Could you check a few things on this model? Use its own coordinates, in mm. A direction names the side the tool comes from. Round coordinates to 2 decimals unless told otherwise and drop trailing zeros. Loops run counter-clockwise (first coordinate to the right, second up) from the corner with the lowest first, then second, coordinate; pieces in that order, holes last. Notation, with made-up numbers: M 7.25,18 L 49.25,18 A15 ccw 49.25,47 Z; hole C -24.75,79.25 d2. An arc over 180 degrees is marked long. Answer in a Markdown table with one row per item.
Autodesk Inventor part; units mm, degrees
ref_plane "YZ Plane" through (0, 0, 0) normal (1, 0, 0) x (0, 1, 0)
ref_plane "XZ Plane" through (0, 0, 0) normal (0, 1, 0) x (-1, 0, 0)
ref_plane "XY Plane" through (0, 0, 0) normal (0, 0, 1) x (1, 0, 0)
sketch "Sketch1" plane through (0, 0, 0) normal (1, 0, 0) x (0, 1, 0)
  line L0 (0, 0) -> (73.993, 0)
  line L1 (0, 130.0359) -> (44.4227, 130.0359)
  line L2 (0, 130.0359) -> (0, 155.2107)
  line L3 (15.8613, 155.2107) -> (44.4227, 155.2107)
  line L4 (44.4227, 155.2107) -> (44.4227, 130.0359)
  line L5 (1.5875, 153.6232) -> (1.5875, 131.6234)
  line L6 (1.5875, 131.6234) -> (42.8352, 131.6234)
  line L7 (42.8352, 131.6234) -> (42.8352, 153.6232)
  line L8 (18.2426, 143.1015) -> (18.2426, 119.3292)
  line L9 (14.2738, 131.6234) -> (14.2738, 130.0359)
  line L10 (22.2113, 131.6234) -> (22.2113, 130.0359)
  line L11 (22.2113, 167.4765) -> (22.2113, 148.4065)
  line L12 (22.2113, 154.417) -> (28.5613, 154.417)
  line L13 (28.5613, 154.417) -> (28.5613, 153.6232)
  line L14 (22.2113, 154.417) -> (15.8613, 154.417)
  line L15 (15.8613, 154.417) -> (15.8613, 155.2107)
  line L16 (42.8352, 153.6232) -> (28.5613, 153.6232)
  line L17 (18.2426, 153.6232) -> (1.5875, 153.6232)
  dimension "d1" = 25.1748
  dimension "d2" = 130.0359
  dimension "d3" = 44.4227
  dimension "d4" = 0
  dimension "d5" = 1.5875
  dimension "d6" = 1.5875
  dimension "d7" = 1.5875
  dimension "d8" = 1.5875
  dimension "d9" = 18.2426
  dimension "d10" = 7.9375
  dimension "d11" = 3.9688
  dimension "d13" = 22.2113
  dimension "d15" = 6.35
  dimension "d16" = 6.35
revolve "Revolution1" add sketch "Sketch1" angle 90 about axis through (0, 0, 0) along (0, 1, 0) contours L10 L6 L7 L16 L13 L12 L11 L3 L4 L1 | L11 L14 L15 L3
equation "\"d2\" = 0.5 * IBDia - 3 * SpWall"
equation "\"d3\" = Wall + 4 * SpWall + BevDriverDia + d1_1"
equation "\"d5\" = Wall"
equation "\"d6\" = Wall"
equation "\"d7\" = Wall"
equation "\"d8\" = Wall"
equation "\"d9\" = 2 * SpWall + 0.5 * BevDriverDia"
equation "\"d10\" = AxelDia + Space"
equation "\"d11\" = 0.5 * Space + 0.5 * AxelDia"
equation "\"d13\" = 0.5 * d3"
equation "\"IDia\" = 266.7"
equation "\"Wall\" = 1.5875"
equation "\"Space\" = 1.5875"
equation "\"SpWall\" = 3.175"
equation "\"AxelDia\" = 6.35"
equation "\"d14\" = 0.5 * Wall"
properties part number "OuterShell_Top_Quarter"
1) I want a section at B-B, the plane x = 32. Please give me the cut outline in (y, z).
Computed:
| item | result |
|---|---|
| outline | M 15.86,151.06 L 28.56,151.06 L 28.56,150.25 L 42.84,150.25 L 42.84,127.67 L 22.21,127.67 L 22.21,126.04 L 44.42,126.04 L 44.42,151.88 L 15.86,151.88 Z |
2) I want a section at C-C, the plane z = 15. Please give me the cut outline in (x, y).
Computed:
| item | result |
|---|---|
| outline | M 129.17,22.21 L 130.77,22.21 L 130.77,42.84 L 152.89,42.84 L 152.89,28.56 L 153.69,28.56 L 153.69,15.86 L 154.48,15.86 L 154.48,44.42 L 129.17,44.42 Z |
3) Will these pins go through, and if not, where does the flat tip stop? P1, Ø2, axis at y = 33, z = 27, coming from the -X side; P2, Ø1.5, axis at y = 23.5, z = 77, coming from the +X side; P3, Ø8, axis at y = 20, z = 136.5, coming from the -X side.
Computed:
| item | result |
|---|---|
| P1 | stops at x = 126.99 |
| P2 | stops at x = 135.19 |
| P3 | stops at x = 64.07 |
4) I need wall thicknesses on line 1 (Y direction, x = 38, z = 131); line 2 (Z direction, x = 64, y = 29); line 3 (X direction, y = 27.5, z = 31.5). Which ranges of each line are inside material? Lowest first, please.
Computed:
| item | result |
|---|---|
| line 1 | y = 42.84 to 44.42 |
| line 2 | z = 113.2 to 115.02, 139.66 to 141.4 |
| line 3 | x = 126.16 to 127.8, 151.17 to 151.98 |
5) Which directions (+Z, -Z, +X, -X, +Y, -Y) give clear straight access to the entire face, cutting with the end or side of a thin tool? Please do faces 5 (the face through (109.816, 35.598, 107.427)), 6 (the face through (90.933, 33.472, 92.955)).
Computed:
| item | result |
|---|---|
| face 5 | -Y |
| face 6 | -Z, -X, +Y, -Y |
6) I want a section at A-A, the plane y = 24.5. Please give me the cut outline in (x, z), plus the area to 3 significant figures.
Computed:
| item | result |
|---|---|
| outline | M 0,130.04 A130.04 cw 130.04,0 L 131.62,0 A131.62 ccw 0,131.62 Z; M 0,154.42 A154.42 cw 154.42,0 L 155.21,0 A155.21 ccw 0,155.21 Z |
| area | 519 mm² |
7) If we mould it in two halves opening along X, with no side actions, what happens to faces 1 (the face through (0, 44, 144)), 2 (the face through (108.54, 30.34, 110.95)), 3 (the face through (107.982, 22.3, 110.383)), 4 (the face through (100, 22.211, 85))? For each: released by +X, released by -X, zero draft, split by the parting line, or undercut.
Computed:
| item | result |
|---|---|
| face 1 | released by -X |
| face 2 | released by +X |
| face 3 | undercut |
| face 4 | zero draft |
8) I want a section at D-D, the plane y = 36.75. Please give me the cut outline in (x, z).
Computed:
| item | result |
|---|---|
| outline | M 0,130.04 A130.04 cw 130.04,0 L 131.62,0 A131.62 ccw 0,131.62 Z; M 0,153.62 A153.62 cw 153.62,0 L 155.21,0 A155.21 ccw 0,155.21 Z |
